from build123d import *

# Parameters (mm, degrees)
SKETCH_1_R          = 9.985
EXTRUDE_1_DEPTH     = 4
SKETCH_2_R          = 11.5
EXTRUDE_2_DEPTH     = 3
SKETCH_3_R          = 21
SKETCH_3_R_2        = 1.5
EXTRUDE_3_DEPTH     = 2
SKETCH_4_R          = 6
CUT_EXTRUDE_1_DEPTH = 32.032241298
FILLET_1_R          = 1.5


with BuildPart() as part:
    # 草图1 → 凸台-拉伸1 (new body)
    with BuildSketch(Plane.XY):
        Circle(SKETCH_1_R)
    extrude(amount=EXTRUDE_1_DEPTH)

    # 草图2 → 凸台-拉伸2 (add)
    with BuildSketch(Plane.XY.offset(4)):
        Circle(SKETCH_2_R)
    extrude(amount=EXTRUDE_2_DEPTH)

    # 草图3 → 凸台-拉伸3 (add)
    with BuildSketch(Plane.XY.offset(7)):
        Circle(SKETCH_3_R)
        with Locations((0, 16)):
            Circle(SKETCH_3_R_2, mode=Mode.SUBTRACT)
        with Locations((13.856406461, 8)):
            Circle(SKETCH_3_R_2, mode=Mode.SUBTRACT)
        with Locations((13.856406461, -8)):
            Circle(SKETCH_3_R_2, mode=Mode.SUBTRACT)
        with Locations((0, -16)):
            Circle(SKETCH_3_R_2, mode=Mode.SUBTRACT)
        with Locations((-13.856406461, -8)):
            Circle(SKETCH_3_R_2, mode=Mode.SUBTRACT)
        with Locations((-13.856406461, 8)):
            Circle(SKETCH_3_R_2, mode=Mode.SUBTRACT)
    extrude(amount=EXTRUDE_3_DEPTH)

    # 草图4 → 切除-拉伸1 (cut, through all)
    with BuildSketch(Plane(origin=(0, 0, 0), x_dir=(-1, 0, 0), z_dir=(0, 0, -1))):
        Circle(SKETCH_4_R)
    extrude(amount=-CUT_EXTRUDE_1_DEPTH, mode=Mode.SUBTRACT)

    # 圆角1
    fillet_1_edges = [part.edges().sort_by_distance(p)[0] for p in [
        (-11.5, 0, 7),
    ]]
    fillet(fillet_1_edges, radius=FILLET_1_R)


solid = part.part
Read the model definition and answer for the solid it produces. Units are mm, in the model's axes. A direction names the side the tool comes from. Give positions to 0.01 mm unless a question says otherwise; leave off trailing zeros. Write each loop counter-clockwise with the first axis right and the second up, starting at its lowest first coordinate (ties: lowest second). Pieces come first, ordered by that corner, then holes. Notation, with made-up numbers: (3, 68.5) - (19, 68.5) arc R13 ccw to (19, 76.5) - close; hole circle Ø9 at (-38, -11.5). An arc over 180 degrees is marked (long way). Answer in a Markdown table with one row per item. Add a question column.
Item 1: Flat-ended cylindrical pins translate along their axes: P1, Ø4, axis at x = 14, y = -4.5, coming from the -Z side; P2, Ø2, axis at x = -9.5, z = 4, coming from the -Y side. Find the tip coordinate at first contact, or state that the pin passes through.
Item 2: Section A-A, the plane y = 0 is taken. Write down the section's boundary in (x, z) (3 decimals).
Item 3: Find the intervals of material crossed by L1, parallel to Y at x = 0, z = 2.5 (3 decimals); L2, parallel to Z at x = 0, y = -13.5; L3, parallel to Y at x = -2.5, z = 2.25, in increasing order.
Item 4: Section B-B, the plane z = 8 is taken. Write down the section's boundary in (x, y).
Item 5: Section C-C, the plane x = 13.5 is taken. Write down the section's boundary in (y, z), and give its area (3 significant figures).
Item 6: A tool of negligible diameter and unlimited length cuts with its end or side. For faces 1 (the face through (-1.5, 11.4, 4.7)), 2 (the face through (20.03, 6.31, 7.99)), from which of +Z, -Z, +X, -X, +Y, -Y can it reach the whole face along a straight path? Write none if from no direction.
Item 7: Determine the mould class of faces 3 (the face through (0, -7, 0)), 4 (the face through (-0.325, -17.464, 7.986)), 5 (the face through (-7.92, -6.08, 1.97)) for opening direction X: pulls with the +X half, pulls with the -X half, needs draft (parallel to the pull), parting line crosses it, or undercut.
Item 8: Section D-D, the plane z = 1 is taken. Write down the section's boundary in (x, y) (3 decimals).
Recorded:
| question | item | result |
|---|---|---|
| 1 | P1 | stops at z = 6.97 |
| 1 | P2 | stops at y = -7.75 |
| 2 | outline | (-21, 7) - (-13, 7) arc R1.5 cw to (-11.5, 5.5) - (-11.5, 4) - (-9.985, 4) - (-9.985, 0) - (-6, 0) - (-6, 9) - (-21, 9) - close; (6, 0) - (9.985, 0) - (9.985, 4) - (11.5, 4) - (11.5, 5.5) arc R1.5 cw to (13, 7) - (21, 7) - (21, 9) - (6, 9) - close |
| 3 | L1 | y = -9.985 to -6, 6 to 9.985 |
| 3 | L2 | z = 7 to 9 |
| 3 | L3 | y = -9.67 to -5.45, 5.45 to 9.67 |
| 4 | outline | circle Ø42 at (0, 0); hole circle Ø3 at (-13.86, -8); hole circle Ø3 at (-13.86, 8); hole circle Ø12 at (0, 0); hole circle Ø3 at (0, -16); hole circle Ø3 at (0, 16); hole circle Ø3 at (13.86, -8); hole circle Ø3 at (13.86, 8) |
| 5 | outline | (-16.09, 7) - (-9.46, 7) - (-9.46, 9) - (-16.09, 9) - close; (-6.54, 7) - (6.54, 7) - (6.54, 9) - (-6.54, 9) - close; (9.46, 7) - (16.09, 7) - (16.09, 9) - (9.46, 9) - close |
| 5 | area | 52.7 mm2 |
| 6 | face 1 | -Z |
| 6 | face 2 | +Z, -Z |
| 7 | face 3 | needs draft |
| 7 | face 4 | undercut |
| 7 | face 5 | parting line crosses it |
| 8 | outline | circle Ø19.97 at (0, 0); hole circle Ø12 at (0, 0) |
